The listing builds one solid part. Answer for the finished solid, in the listing's coordinates (mm). A direction names the side the tool comes from. Coordinates: 2 decimals unless noted, no trailing zeros. Order: outer loops, then holes, each group sorted by start corner. A loop starts at its lowest first (then second) coordinate and runs counter-clockwise, first axis right, second up. Notation, with made-up numbers: (81.5, 39) - (126.5, 39) arc R13 ccw to (126.5, 45) - close; hole circle Ø1 at (50.25, 69.5). An arc over 180 degrees is marked (long way). One line per item, written item: value. Start each with the question number.
```python
from build123d import *

# Parameters (mm, degrees)
SKETCH_1_R          = 18
EXTRUDE_1_DEPTH     = 38
SKETCH_2_R          = 11
EXTRUDE_2_DEPTH     = 2
EXTRUDE_START       = 2
SKETCH_3_R          = 11
EXTRUDE_3_DEPTH     = 2
SKETCH_4_R          = 4
EXTRUDE_4_DEPTH     = 18
SKETCH_5_R          = 3
EXTRUDE_5_DEPTH     = 18
SKETCH_6_W          = 9.252434457
SKETCH_6_H          = 4.602247191
CUT_EXTRUDE_1_DEPTH = 15
SKETCH_7_W          = 9.252434457
SKETCH_7_H          = 4.602247191
CUT_EXTRUDE_2_DEPTH = 15
SKETCH_8_R          = 1.5
CUT_EXTRUDE_3_DEPTH = 6
CUT_EXTRUDE_START   = -6
SKETCH_9_R          = 1.5
CUT_EXTRUDE_4_DEPTH = 6


with BuildPart() as part:
    # 草图1 → 凸台-拉伸1 (new body)
    with BuildSketch(Plane(origin=(0, 0, 0), x_dir=(1, 0, 0), z_dir=(0, 1, 0))):
        with Locations(Location((0, 0, 0), (0, 0, 270))):
            Circle(SKETCH_1_R)
    extrude(amount=EXTRUDE_1_DEPTH)

    # 草图2 → 凸台-拉伸2 (add)
    with BuildSketch(Plane(origin=(0, 38, 0), x_dir=(1, 0, 0), z_dir=(0, 1, 0))):
        with Locations(Location((0, 0, 0), (0, 0, 270))):
            Circle(SKETCH_2_R)
    extrude(amount=EXTRUDE_2_DEPTH)

    # 草图3 → 凸台-拉伸3 (add)
    with BuildSketch(Plane.XZ.offset(EXTRUDE_START)):
        with Locations(Location((0, 0, 0), (0, 0, 90))):
            Circle(SKETCH_3_R)
    extrude(amount=-EXTRUDE_3_DEPTH)

    # 草图4 → 凸台-拉伸4 (add)
    with BuildSketch(Plane.XZ.offset(2)):
        with Locations(Location((0, 0, 0), (0, 0, 270))):
            Circle(SKETCH_4_R)
    extrude(amount=EXTRUDE_4_DEPTH)

    # 草图5 → 凸台-拉伸5 (add)
    with BuildSketch(Plane(origin=(0, 40, 0), x_dir=(1, 0, 0), z_dir=(0, 1, 0))):
        with Locations(Location((0, 0, 0), (0, 0, 270))):
            Circle(SKETCH_5_R)
    extrude(amount=EXTRUDE_5_DEPTH)

    # 草图6 → 切除-拉伸1 (cut)
    with BuildSketch(Plane(origin=(0, 58, 0), x_dir=(1, 0, 0), z_dir=(0, 1, 0))):
        with Locations((-0.167790263, 4.301123596)):
            Rectangle(SKETCH_6_W, SKETCH_6_H)
    extrude(amount=-CUT_EXTRUDE_1_DEPTH, mode=Mode.SUBTRACT)

    # 草图7 → 切除-拉伸2 (cut)
    with BuildSketch(Plane.XZ.offset(20)):
        with Locations((-0.167790263, -4.301123596)):
            Rectangle(SKETCH_7_W, SKETCH_7_H)
    extrude(amount=-CUT_EXTRUDE_2_DEPTH, mode=Mode.SUBTRACT)

    # 草图8 → 切除-拉伸3 (cut)
    with BuildSketch(Plane.XZ):
        with Locations(Location((0, 14, 0), (0, 0, 270))):
            Circle(SKETCH_8_R)
        with Locations(Location((14, 0, 0), (0, 0, 270))):
            Circle(SKETCH_8_R)
        with Locations(Location((0, -14, 0), (0, 0, 270))):
            Circle(SKETCH_8_R)
        with Locations(Location((-14, 0, 0), (0, 0, 270))):
            Circle(SKETCH_8_R)
    extrude(amount=-CUT_EXTRUDE_3_DEPTH, mode=Mode.SUBTRACT)

    # 草图9 → 切除-拉伸4 (cut)
    with BuildSketch(Plane(origin=(0, 38, 0), x_dir=(1, 0, 0), z_dir=(0, 1, 0)).offset(CUT_EXTRUDE_START)):
        with Locations(Location((-14, 0, 0), (0, 0, 90))):
            Circle(SKETCH_9_R)
        with Locations(Location((0, 14, 0), (0, 0, 90))):
            Circle(SKETCH_9_R)
        with Locations(Location((14, 0, 0), (0, 0, 90))):
            Circle(SKETCH_9_R)
        with Locations(Location((0, -14, 0), (0, 0, 90))):
            Circle(SKETCH_9_R)
    extrude(amount=CUT_EXTRUDE_4_DEPTH, mode=Mode.SUBTRACT)


solid = part.part
```
(1) Consider probe 1 along X at (y, z) = (36.55, 0); probe 2 along Y at (x, z) = (15.5, 4); probe 3 along Y at (x, z) = (9.5, 3). Determine where each line is inside the solid, lowest interval first.
(2) Flat-ended cylindrical pins translate along their axes: pin 1 Ø3.5 at (x, z) = (0, -14) entering from +Y; pin 2 Ø0.9 at (x, z) = (-14, -0.5) entering from +Y; pin 3 Ø1.3 at (x, y) = (-0.5, 50.5) entering from -Z. Find the tip coordinate at first contact, or state that the pin passes through.
(3) For faces 1 (the face through (0, 32, -14)), 2 (the face through (0, 6, 14)), 3 (the face through (0, 51, -2)), determine the directions among +Z, -Z, +X, -X, +Y, -Y from which every point of the face is accessible in a straight line to the end or side of a thin tool.
(4) The part is cut by section B-B on x = -7. Determine the outline of the cut face in (y, z).
(5) For a pull along X with two mould halves and no side action, classify faces 4 (the face through (0.9, 48.87, 2.86)), 5 (the face through (0, -13, -2)), 6 (the face through (-14.45, 34.96, -1.43)), 7 (the face through (0.07, 2.96, 15.5)) as pulls with the +X half, pulls with the -X half, needs draft (parallel to the pull), parting line crosses it, or undercut.
(6) The part is cut by section A-A on z = -5. Determine the outline of the cut face in (x, y), plus the area to 3 significant figures.
(7) The part is cut by section C-C on y = -8.5. Determine the outline of the cut face in (x, z).
Completed:
1. probe 1: x = -18 to -15.5, -12.5 to 12.5, 15.5 to 18
1. probe 2: y = 0 to 38
1. probe 3: y = -2 to 40
2. pin 1: stops at y = 38
2. pin 2: stops at y = 32
2. pin 3: stops at z = -2
3. face 1: +Y
3. face 2: -Y
3. face 3: -Z, +X, -X, +Y
4. outline: (-2, -8.49) - (0, -8.49) - (0, -16.58) - (38, -16.58) - (38, -8.49) - (40, -8.49) - (40, 8.49) - (38, 8.49) - (38, 16.58) - (0, 16.58) - (0, 8.49) - (-2, 8.49) - close
5. face 4: parting line crosses it
5. face 5: needs draft
5. face 6: undercut
5. face 7: undercut
6. outline: (-17.29, 0) - (-9.8, 0) - (-9.8, -2) - (9.8, -2) - (9.8, 0) - (17.29, 0) - (17.29, 38) - (9.8, 38) - (9.8, 40) - (-9.8, 40) - (-9.8, 38) - (-17.29, 38) - close
6. area: 1,390 mm2
7. outline: (-3.46, -2) - (3.46, -2) arc R4 ccw (long way) to start
